The model under review builds one solid part; all positions refer to its coordinate system, in mm. A direction names the side the tool comes from. Coordinates: 2 decimals unless noted, no trailing zeros. Loops run counter-clockwise (first coordinate to the right, second up) from the corner with the lowest first, then second, coordinate; pieces in that order, holes last. Notation, with made-up numbers: M 21,80 L 29,80 A13 ccw 29,88 Z; hole C 12,21.25 d9. An arc over 180 degrees is marked long. Use CSV: the item, a comma, the result in double quotes. Start each with the question number.
1. Add section D-D, the plane y = -80. Write out the cut boundary in (x, z).
2. Clearance check with flat-ended pins moving along their axes: P1, Ø6, axis at x = -56.5, z = 144, coming from the -Y side; P2, Ø1.5, axis at y = -77, z = 2, coming from the +X side; P3, Ø10, axis at x = -177.8, z = 25.146, coming from the +Y side; P4, Ø0.9, axis at y = -79.5, z = 1, coming from the -X side. State where each tip first meets the part, or that it passes through.
3. Add section C-C, the plane z = 134.5. Write out the cut boundary in (x, y), then the cut area to 3 significant figures.
4. Draft analysis for pull direction Z (two halves, no side actions). For faces 4 (the cylindrical face through (-180.948, 1.503, 158.083)), 5 (the flat face through (-100, 3.048, 87)), 6 (the flat face through (-101.9, -96.2, 1.524)), 7 (the cylindrical face through (-100.178, 1.215, 1.738)), state which applies: +Z half, -Z half, draft (parallel to the pull), parting line (faces both ways), or undercut.
5. Add section A-A, the plane x = -101.6. Write out the cut boundary in (y, z), then the cut area to 3 significant figures.
6. Add section B-B, the plane x = -177.8. Write out the cut boundary in (y, z).
7. Tool access review of faces 1 (the cylindrical face through (-199.38, -12.13, 1.5)), 2 (the flat face through (-100, -49, 3.048)), 3 (the cylindrical face through (-91.36, -76.14, 2.3)): name each direction out of +Z, -Z, +X, -X, +Y, -Y from which nothing blocks a thin tool from reaching the whole face with its end or side.
8. For L1, parallel to Z at x = -25.4, y = 2.2; L2, parallel to Y at x = -101, z = 2; L3, parallel to Z at x = -177.8, y = 2, list the stretches that pass through material, from the lowest coordinate up.
Autodesk Inventor part; units mm, degrees
ref_plane "YZ Plane" through (0, 0, 0) normal (1, 0, 0) x (0, 1, 0)
ref_plane "XZ Plane" through (0, 0, 0) normal (0, 1, 0) x (-1, 0, 0)
ref_plane "XY Plane" through (0, 0, 0) normal (0, 0, 1) x (1, 0, 0)
sketch "Sketch1" plane through (0, 0, 0) normal (0, 1, 0) x (-1, 0, 0)
  line L0 (0, 0) -> (203.2, 0)
  line L1 (203.2, 0) -> (203.2, 165.1)
  line L2 (203.2, 165.1) -> (0, 165.1)
  line L3 (0, 165.1) -> (0, 0)
  dimension "d0" = 203.2
  dimension "d1" = 165.1
extrude "Plate2" add sketch "Sketch1" along normal blind 3.048
sketch "Sketch4" plane through (0, 3.048, 3.048) normal (0, 0, -1) x (-1, 0, 0)
  line L0 (203.2, 0) -> (0, 0)
  line L1 (0, 0) -> (0, -127)
  line L2 (0, -127) -> (203.2, -127)
  line L3 (203.2, -127) -> (203.2, 0)
edge flange "Flange1" height 127 angle 90 thickness 3.048 bend radius 3.048 thickness toward (0, 0, -1) relief straight relief width 3.048 relief depth 1.524 edges at (-101.6, 0, 0) wall of the first edge with corners at (-203.2, 3.048, 3.048) (0, 3.048, 3.048) (0, -123.952, 3.048) (-203.2, -123.952, 3.048)
bend "Bend1"
corner "Corner1"
sketch "Sketch5" plane through (0, 3.048, 0) normal (0, 1, 0) x (1, 0, 0)
  line L0 (0, -6.096) -> (-203.2, -6.096)
  line L1 (-203.2, -165.1) -> (-203.2, -6.096)
  line L2 (0, -6.096) -> (0, -165.1)
  point P0 (0, 0)
  point P1 (-177.8, -25.146)
  point P2 (-25.4, -25.146)
  point P3 (-25.4, -158.496)
  point P4 (-177.8, -158.496)
  dimension "d27" = 25.4
  dimension "d28" = 25.4
  dimension "d29" = 19.05
  dimension "d30" = 133.35
hole "Hole2" at (-177.8, 3.048, 25.146) at (-25.4, 3.048, 25.146) at (-25.4, 3.048, 158.496) at (-177.8, 3.048, 158.496) direction (0, -1, 0) diameter 6.35 end through all
sketch "Sketch6" plane through (0, -123.952, 0) normal (0, 0, -1) x (-1, 0, 0)
  line L0 (203.2, 120.904) -> (0, 120.904)
  line L1 (0, 0) -> (0, 120.904)
  line L2 (203.2, 0) -> (0, 0)
  line L3 (203.2, 120.904) -> (203.2, 0)
  line L4 (50.8, 120.904) -> (152.4, 120.904)
  line L5 (152.4, 70.104) -> (152.4, 25.4)
  line L6 (127, 0) -> (76.2, 0)
  line L7 (50.8, 25.4) -> (50.8, 70.104)
  arc A0 (50.8, 25.4) -> (76.2, 0) centre (76.2, 25.4) ccw
  arc A1 (127, 0) -> (152.4, 25.4) centre (127, 25.4) ccw
  line L8 (12.7, 108.204) -> (12.7, 108.204)
  line L9 (0, 0) -> (0, 108.204)
  line L10 (0, 0) -> (76.2, 0)
  line L11 (203.2, 0) -> (127, 0)
  line L12 (190.5, 108.204) -> (190.5, 108.204)
  line L13 (203.2, 108.204) -> (203.2, 0)
  arc A2 (50.8, 70.104) -> (12.7, 108.204) centre (12.7, 70.104) ccw
  arc A3 (190.5, 108.204) -> (152.4, 70.104) centre (190.5, 70.104) ccw
  line L14 (0, 120.904) -> (0, 120.904)
  line L15 (203.2, 120.904) -> (203.2, 120.904)
  arc A4 (190.5, 108.204) -> (203.2, 120.904) centre (190.5, 120.904) ccw
  arc A5 (0, 120.904) -> (12.7, 108.204) centre (12.7, 120.904) ccw
  point P0 (0, 123.952)
  point P1 (152.4, 0)
  point P2 (50.8, 0)
  dimension "d38" = 101.6
  dimension "d40" = 50.8
  dimension "d41" = 50.8
  dimension "d42" = 25.4
  dimension "d43" = 12.7
  dimension "d44" = 38.1
  dimension "d47" = 12.7
extrude "Extrusion2" cut sketch "Sketch6" against normal through all contours L3 L2 A1 L5 A3 A4 | A5 A2 L7 A0 L2 L1
sketch "Sketch8" plane through (-203.2, -3.048, 3.048) normal (0, 0, 1) x (1, 0, 0)
  line L0 (76.2, -120.904) -> (127, -120.904)
  line L1 (152.4, -95.504) -> (152.4, -50.8)
  line L2 (50.8, -50.8) -> (50.8, -95.504)
  circle A0 centre (101.6, -89.154) radius 19.05
  point P0 (203.2, 3.048)
  dimension "d53" = 38.1
  dimension "d54" = 50.8
  dimension "d55" = 50.8
  dimension "d56" = 31.75
extrude "Extrusion3" cut sketch "Sketch8" against normal blind 1.524
sketch "Sketch9" plane through (-101.6, -92.202, 1.524) normal (0, 0, 1) x (1, 0, 0)
  circle A0 centre (0, 0) radius 19.05
  circle A1 centre (0, 0) radius 3.81
  point P0 (101.6, 92.202)
  dimension "d59" = 7.62
extrude "Extrusion4" cut sketch "Sketch9" against normal through all contours A1
equation "\"d40\" = d41"
equation "\"d17\" = BendReliefWidth"
equation "\"d18\" = BendReliefDepth"
equation "\"d19\" = MinimumRemnant"
equation "\"d20\" = BendRadius"
equation "\"d23\" = BendRadius"
equation "\"d24\" = CornerReliefSize"
equation "\"d25\" = GapSize"
equation "\"d26\" = JacobiRadiusSize"
equation "\"BendRadius\" = Thickness"
equation "\"BendReliefWidth\" = Thickness"
equation "\"BendReliefDepth\" = 0.5 * Thickness"
equation "\"CornerReliefSize\" = 4 * Thickness"
equation "\"MinimumRemnant\" = 2 * Thickness"
equation "\"TransitionRadius\" = BendRadius"
equation "\"JacobiRadiusSize\" = Thickness"
equation "\"GapSize\" = Thickness"
equation "\"d15\" = BendRadius"
equation "\"d16\" = BendRadius"
properties part number "backplate"
Computed:
1,outline,"M -152.4,0 L -50.8,0 L -50.8,3.05 L -86.97,3.05 L -86.97,1.52 L -116.23,1.52 L -116.23,3.05 L -152.4,3.05 Z"
2,P1,"stops at y = 0"
2,P2,"stops at x = -50.8"
2,P3,"stops at y = 3.05"
2,P4,"stops at x = -152.4"
3,outline,"M -203.2,0 L 0,0 L 0,3.05 L -203.2,3.05 Z"
3,area,"619 mm^2"
4,face 4,"undercut"
4,face 5,"draft"
4,face 6,"+Z half"
4,face 7,"-Z half"
5,outline,"M -123.95,0 L -96.01,0 L -96.01,1.52 L -111.25,1.52 L -111.25,3.05 L -123.95,3.05 Z; M -88.39,0 L -3.05,0 A6.1 ccw 3.05,6.1 L 3.05,165.1 L 0,165.1 L 0,6.1 A3.05 cw -3.05,3.05 L -73.15,3.05 L -73.15,1.52 L -88.39,1.52 Z"
5,area,"805 mm^2"
6,outline,"M -17.93,0 L -3.05,0 A6.1 ccw 3.05,6.1 L 3.05,21.97 L 0,21.97 L 0,6.1 A3.05 cw -3.05,3.05 L -17.93,3.05 Z; M 0,28.32 L 3.05,28.32 L 3.05,155.32 L 0,155.32 Z; M 0,161.67 L 3.05,161.67 L 3.05,165.1 L 0,165.1 Z"
7,face 1,"+Z, -Z, -X, -Y"
7,face 2,"+Z, +X, -X, -Y"
7,face 3,"+Z"
8,L1,"z = 2.99 to 21.97, 28.32 to 155.32, 161.67 to 165.1"
8,L2,"y = -123.95 to -111.24, -73.16 to 1.47"
8,L3,"z = 2.68 to 21.97, 28.32 to 155.32, 161.67 to 165.1"
